Could you check a few things on this model? Use its own coordinates, in mm. A direction names the side the tool comes from. Round coordinates to 2 decimals unless told otherwise and drop trailing zeros. Write each loop counter-clockwise with the first axis right and the second up, starting at its lowest first coordinate (ties: lowest second). Pieces come first, ordered by that corner, then holes. Notation, with made-up numbers: (8.25, 42) - (40.25, 42) arc R29 ccw to (40.25, 79) - close; hole circle Ø1 at (85.25, 66). An arc over 180 degrees is marked (long way). Put each result on its own line as item: value.
from build123d import *

# Parameters (mm, degrees)
BOSS_EXTRUDE1_DEPTH   = 200
BOSS_EXTRUDE1_2_DEPTH = 200
SKETCH2_R             = 2.4
BOSS_EXTRUDE2_DEPTH   = 10
SKETCH3_R             = 2.4
BOSS_EXTRUDE3_DEPTH   = 10
SKETCH4_W             = 46
SKETCH4_H             = 10
BOSS_EXTRUDE4_DEPTH   = 10
BOSS_EXTRUDE5_START   = 3.5
SKETCH5_W             = 33
SKETCH5_H             = 10
SKETCH5_R             = 2.535
BOSS_EXTRUDE5_DEPTH   = 4


with BuildPart() as part:
    # Sketch1 → Boss-Extrude1 (new body)
    with BuildSketch(Plane.XY):
        Polygon((4, 10), (7, 7), (7, 0), (0, 0), (0, 10), align=None)
    extrude(amount=BOSS_EXTRUDE1_DEPTH)

    # Sketch3 → Boss-Extrude3 (add)
    with BuildSketch(Plane.ZY):
        with Locations((100, 5)):
            Circle(SKETCH3_R)
    extrude(amount=BOSS_EXTRUDE3_DEPTH)



with BuildPart() as body_2:
    # Sketch1 → Boss-Extrude1 2 (new body)
    with BuildSketch(Plane.XY):
        Polygon((39, 0), (39, 7), (42, 10), (46, 10), (46, 0), align=None)
    extrude(amount=BOSS_EXTRUDE1_2_DEPTH)

    # Sketch2 → Boss-Extrude2 (add)
    with BuildSketch(Plane(origin=(46, 0, 0), x_dir=(0, 0, -1), z_dir=(1, 0, 0))):
        with Locations((-100, 5)):
            Circle(SKETCH2_R)
    extrude(amount=BOSS_EXTRUDE2_DEPTH)


with BuildPart() as part_1:
    add(part.part)

    add(body_2.part)  # Boss-Extrude4 merges body 2
    # Sketch4 → Boss-Extrude4 (add)
    with BuildSketch(Plane.XZ):
        with Locations((23, 195)):
            Rectangle(SKETCH4_W, SKETCH4_H)
    boss_extrude4 = extrude(amount=-BOSS_EXTRUDE4_DEPTH)

    # Mirror3: Boss-Extrude4 across plane
    add(boss_extrude4.mirror(Plane(origin=(0, 0, 100), x_dir=(1, 0, 0), z_dir=(0, 0, -1))))

    # Sketch5 → Boss-Extrude5 (add)
    with BuildSketch(Plane(origin=(23, 0, 0), x_dir=(0, 0, -1), z_dir=(1, 0, 0)).offset(BOSS_EXTRUDE5_START)):
        with Locations((-206.5, 5)):
            Rectangle(SKETCH5_W, SKETCH5_H)
        with Locations((-218, 5)):
            Circle(SKETCH5_R, mode=Mode.SUBTRACT)
    boss_extrude5 = extrude(amount=BOSS_EXTRUDE5_DEPTH)

    # Mirror4: Boss-Extrude5 across plane
    add(boss_extrude5.mirror(Plane(origin=(23, 0, 0), x_dir=(0, 0, 1), z_dir=(1, 0, 0))))


solid = part_1.part
(1) Imagine slicing it at C-C, the plane x = 13. List the corners of the cut face in (y, z) for me.
Values found:
outline: (0, 0) - (10, 0) - (10, 10) - (0, 10) - close; (0, 190) - (10, 190) - (10, 200) - (0, 200) - close
(2) If we mould it in two halves opening along X, with no side actions, what happens to faces 6 (the face through (0, 7.2, 98.6)), 7 (the face through (28, 5, 223)), 8 (the face through (19.5, 5, 212)), 9 (the face through (46, 2.8, 98.6))? For each: pulls with the +X half, pulls with the -X half, needs draft (parallel to the pull), parting line crosses it, or undercut.
Values found:
face 6: pulls with the -X half
face 7: needs draft
face 8: undercut
face 9: pulls with the +X half
(3) For faces 1 (the face through (26.5, 5, 212)), 2 (the face through (50.93, 4.081, 97.783)), 3 (the face through (15.5, 5, 212)), 4 (the face through (38, 5, 200)), 5 (the face through (7, 4, 99)), which set-ups out of +Z, -Z, +X, -X, +Y, -Y let a thin tool reach every point of the face, with its end or its side?
Values found:
face 1: +Z, +Y, -Y
face 2: +X
face 3: +Z, -X, +Y, -Y
face 4: +Z, +X, +Y, -Y
face 5: +Y, -Y
(4) Please list where these lines run through material, in increasing order: probe 1 along X at (y, z) = (7.25, 206); probe 2 along X at (y, z) = (1, 87.5); probe 3 along Y at (x, z) = (18, 218) (3 decimals). Write a range as from..to.
Values found:
probe 1: x = 15.5..19.5, 26.5..30.5
probe 2: x = 0..7, 39..46
probe 3: y = 0..2.465, 7.535..10
(5) Imagine slicing it at A-A, the plane y = 5. Give the number of separate pieces and of enclosed holes in the cut face, then the cut area to 3 significant figures.
Values found:
separate pieces: 3
enclosed holes: 1
area: 3,680 mm^2
(6) Imagine slicing it at B-B, the plane z = 218. List the corners of the cut face in (x, y) for me (3 decimals).
Values found:
outline: (15.5, 0) - (19.5, 0) - (19.5, 2.465) - (15.5, 2.465) - close; (15.5, 7.535) - (19.5, 7.535) - (19.5, 10) - (15.5, 10) - close; (26.5, 0) - (30.5, 0) - (30.5, 2.465) - (26.5, 2.465) - close; (26.5, 7.535) - (30.5, 7.535) - (30.5, 10) - (26.5, 10) - close
(7) Imagine slicing it at D-D, the plane z = 100. List the corners of the cut face in (x, y) for me.
Values found:
outline: (-10, 2.6) - (0, 2.6) - (0, 0) - (7, 0) - (7, 7) - (4, 10) - (0, 10) - (0, 7.4) - (-10, 7.4) - close; (39, 0) - (46, 0) - (46, 2.6) - (56, 2.6) - (56, 7.4) - (46, 7.4) - (46, 10) - (42, 10) - (39, 7) - close
(8) I'm going to push flat-ended pins straight in: pin 1 (1.5 mm diameter, centred on y = 3.5, z = 110.5, fed in from -X); pin 2 (2 mm diameter, centred on x = 21.5, y = 3, fed in from +Z); pin 3 (5.5 mm diameter, centred on y = 2, z = 132.5, fed in from +X). Where does each tip first touch, or does it pass through?
Values found:
pin 1: stops at x = 0
pin 2: stops at z = 200
pin 3: stops at x = 46
